Here's how the part is built. I have some questions about the finished solid (model axes, mm). Face numbers are marked on the shaded views. A direction names the side the tool comes from. Give positions to 0.01 mm unless a question says otherwise; leave off trailing zeros. Order: outer loops, then holes, each group sorted by start corner. A loop starts at its lowest first (then second) coordinate and runs counter-clockwise, first axis right, second up.
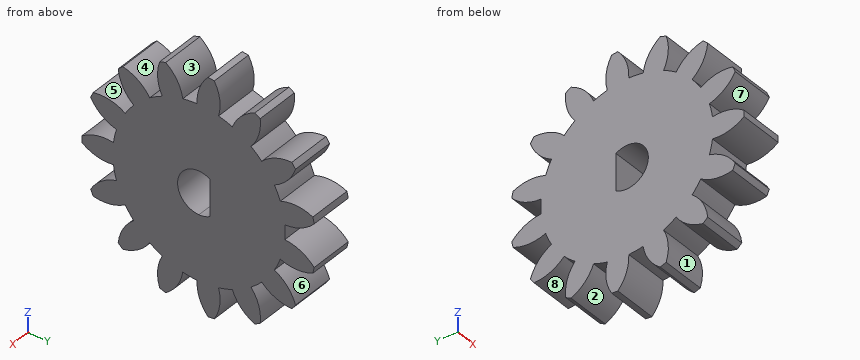
from build123d import *

# Parameters (mm, degrees)
BASPROSKE_W        = 6.35
BASPROSKE_H        = 17
TOOTHCUT_DEPTH     = 25.86609137
TEETHCUTS_COUNT    = 15
TEETHCUTS_ANGLE    = 336
BORSKE_R           = 0.4
BORE_DEPTH         = 50.0000508
CUT_EXTRUDE1_DEPTH = 10


with BuildPart() as part:
    # BasProSke → Base-Revolve (revolve)
    with BuildSketch(Plane(origin=(0, 0, 0), x_dir=(1, 0, 0), z_dir=(0, 1, 0)), mode=Mode.PRIVATE) as base_revolve_sk:
        with Locations((3.175, 8.5)):
            Rectangle(BASPROSKE_W, BASPROSKE_H)
    revolve(base_revolve_sk.sketch.rotate(Axis((-10, 0, 0), (1, 0, 0)), 180), axis=Axis((-10, 0, 0), (1, 0, 0)))

    # TooCutSke → ToothCut (cut, through all)
    with BuildSketch(Plane(origin=(0, 0, 0), x_dir=(0, 0, -1), z_dir=(1, 0, 0))):
        with BuildLine():
            ThreePointArc((1.050056448, 12.454813626), (0, 12.499), (-1.050056448, 12.454813626))
            ThreePointArc((-1.050056448, 12.454813626), (-1.638118106, 14.809604533), (-3.110934279, 16.73876737))
            ThreePointArc((-3.110934279, 16.73876737), (0, 17.0254), (3.110934279, 16.73876737))
            ThreePointArc((3.110934279, 16.73876737), (1.638118106, 14.809604533), (1.050056448, 12.454813626))
        make_face()
    toothcut = extrude(amount=TOOTHCUT_DEPTH, mode=Mode.SUBTRACT)

    # TeethCuts: ToothCut ×15 about axis
    teethcuts_axis = Axis((-10, 0, 0), (1, 0, 0))
    for i in range(1, TEETHCUTS_COUNT):
        add(toothcut.rotate(teethcuts_axis, i * TEETHCUTS_ANGLE / (TEETHCUTS_COUNT - 1)), mode=Mode.SUBTRACT)

    # BorSke → Bore (cut, symmetric)
    with BuildSketch(Plane(origin=(0, 0, 0), x_dir=(0, 0, -1), z_dir=(1, 0, 0))):
        with Locations(Location((0, 0, 0), (0, 0, 180))):
            Circle(BORSKE_R)
    extrude(amount=BORE_DEPTH, both=True, mode=Mode.SUBTRACT)

    # Sketch1 → Cut-Extrude1 (cut)
    with BuildSketch(Plane(origin=(6.35, 0, 0), x_dir=(0, 0, -1), z_dir=(1, 0, 0))):
        with BuildLine():
            Line((2.655183609, 1.6), (-2.655183609, 1.6))
            ThreePointArc((-2.655183609, 1.6), (-0.830340536, -2.986726401), (3.1, 0))
            ThreePointArc((3.1, 0), (2.986726401, 0.830340536), (2.655183609, 1.6))
        make_face()
    extrude(amount=-CUT_EXTRUDE1_DEPTH, mode=Mode.SUBTRACT)


solid = part.part
Q1. I need wall thicknesses on L1, parallel to Y at x = 3.25, z = 0; L2, parallel to Y at x = 0.75, z = 15.5; L3, parallel to Z at x = 1.5, y = 0.5. Which ranges of each line are inside material? Lowest first, please.
Filled sheet:
L1: y = -17 to -3.1, 1.6 to 12.5
L2: y = -5.84 to -3.9, 0.33 to 2.82
L3: z = -15.82 to -3.06, 3.06 to 15.82
Q2. If we section it at B-B on y = 6: List the corners of the cut face in (x, z) for me.
Filled sheet:
outline: (0, -13.43) - (6.35, -13.43) - (6.35, 13.43) - (0, 13.43) - close
Q3. If we section it at A-A on z = 0: List the corners of the cut face in (x, y) for me, plus the area to 3 significant figures.
Filled sheet:
outline: (0, -17) - (6.35, -17) - (6.35, -3.1) - (0, -3.1) - close; (0, 1.6) - (6.35, 1.6) - (6.35, 12.5) - (0, 12.5) - close
area: 157 mm2
Q4. For the marked faces 4, 5, 6, 7 and 8, which set-ups out of +Z, -Z, +X, -X, +Y, -Y let a thin tool reach every point of the face, with its end or its side?
Filled sheet:
face 4: +Z, +X, -X
face 5: +X, -X
face 6: +X, -X, +Y
face 7: +X, -X, -Y
face 8: -Z, +X, -X
Q5. Thinking about a two-plate mould opening in Z: for the marked faces 1, 2 and 3, which applies, released by +Z, released by -Z, zero draft, split by the parting line, or undercut?
Filled sheet:
face 1: undercut
face 2: released by -Z
face 3: released by +Z
Q6. I'm going to push flat-ended pins straight in: P1, Ø2, axis at x = 3.5, z = 1.5, coming from the +Y side; P2, Ø1.5, axis at x = 3.5, y = -10, coming from the -Z side; P3, Ø2, axis at x = 2.5, z = -1.5, coming from the -Y side. Where does each tip first touch, or does it pass through?
Filled sheet:
P1: stops at y = 16.13
P2: stops at z = -12.87
P3: stops at y = -16.94
Q7. If we section it at C-C on y = -4: List the corners of the cut face in (x, z) for me.
Filled sheet:
outline: (0, -15.61) - (6.35, -15.61) - (6.35, 15.61) - (0, 15.61) - close
